from build123d import *

# Parameters (mm, degrees)
SKETCH_W        = 106.5
SKETCH_H        = 150
PAD_DEPTH       = 5
SKETCH001_W     = 5
SKETCH001_H     = 15.5
POCKET_DEPTH    = 5
FILLET_R        = 0.4
POCKET001_DEPTH = 5


with BuildPart() as part:
    # Sketch → Pad (new body)
    with BuildSketch(Plane.XY):
        Rectangle(SKETCH_W, SKETCH_H)
    extrude(amount=PAD_DEPTH)

    # Sketch001 (on Face6 of Pad) → Pocket (cut)
    with BuildSketch(Plane.XY.offset(5)):
        with Locations((-50.75, 67.25)):
            Rectangle(SKETCH001_W, SKETCH001_H)
        with Locations((50.75, 67.25)):
            Rectangle(SKETCH001_W, SKETCH001_H)
        with Locations((50.75, -67.25)):
            Rectangle(SKETCH001_W, SKETCH001_H)
        with Locations((-50.75, -67.25)):
            Rectangle(SKETCH001_W, SKETCH001_H)
    extrude(amount=-POCKET_DEPTH, mode=Mode.SUBTRACT)

    # Fillet
    fillet_edges = [part.edges().sort_by_distance(p)[0] for p in [
        (-48.25, 75, 2.5),
        (-48.25, 59.5, 2.5),
        (-53.25, 59.5, 2.5),
        (48.25, 75, 2.5),
        (48.25, 59.5, 2.5),
        (53.25, 59.5, 2.5),
        (53.25, -59.5, 2.5),
        (48.25, -59.5, 2.5),
        (48.25, -75, 2.5),
        (-48.25, -75, 2.5),
        (-48.25, -59.5, 2.5),
        (-53.25, -59.5, 2.5),
        (-48.25, 67.25, 5),
        (-50.75, 59.5, 5),
        (-53.25, 0, 5),
        (-50.75, -59.5, 5),
        (-48.25, -67.25, 5),
        (0, -75, 5),
        (48.25, -67.25, 5),
        (50.75, -59.5, 5),
        (53.25, 0, 5),
        (50.75, 59.5, 5),
        (48.25, 67.25, 5),
        (0, 75, 5),
    ]]
    fillet(fillet_edges, radius=FILLET_R)

    # Sketch002 (on Face29 of Fillet) → Pocket001 (cut)
    with BuildSketch(Plane.XY.offset(5)):
        with BuildLine():
            ThreePointArc((-40, -40), (-25, -55), (-10, -40))
            Line((-10, -40), (-10, 40))
            ThreePointArc((-10, 40), (-25, 55), (-40, 40))
            Line((-40, -40), (-40, 40))
        make_face()
        with BuildLine():
            ThreePointArc((10, -40), (25, -55), (40, -40))
            Line((40, -40), (40, 40))
            ThreePointArc((40, 40), (25, 55), (10, 40))
            Line((10, -40), (10, 40))
        make_face()
    extrude(amount=-POCKET001_DEPTH, mode=Mode.SUBTRACT)


solid = part.part
Design review of the part built by this model. Coordinates are the model's own, in mm. A direction names the side the tool comes from. Coordinates: 2 decimals unless noted, no trailing zeros. Order: outer loops, then holes, each group sorted by start corner. A loop starts at its lowest first (then second) coordinate and runs counter-clockwise, first axis right, second up.
Item 1: For faces 4 (the flat face through (48.25, 67, 2)), 5 (the flat face through (-48.25, 67, 2)), 6 (the flat face through (-10, -1, 3)), 7 (the flat face through (-51, -59.5, 2)), list the 3-axis set-ups (+Z, -Z, +X, -X, +Y, -Y) from which the entire face can be reached by the end or side of a thin tool; tool diameter is ignored.
Item 2: Take a section at A-A, the plane y = -16. Write out the cut boundary in (x, z), then the cut area to 3 significant figures.
Item 3: The part is to be moulded in two halves that separate along X. For faces 1 (the flat face through (-53.25, -1, 2)), 2 (the cylindrical face through (25, 55, 3)), 3 (the flat face through (-1, 75, 2)), say which applies: pulls with the +X half, pulls with the -X half, needs draft (parallel to the pull), parting line crosses it, or undercut.
Item 4: Take a section at B-B, the plane x = 25. Write out the cut boundary in (y, z).
Item 5: For pin 1 Ø2 at (x, z) = (50, 1) entering from +Y; pin 2 Ø2.5 at (y, z) = (66.5, 3) entering from +X; pin 3 Ø1.3 at (x, z) = (51, 1) entering from -Y, all flat-tipped, find the tip position at first contact; note any pin that passes through.
Item 6: Take a section at C-C, the plane z = 1.2. Count the separate pieces of the cut face and the enclosed holes in it, then the cut area to 3 significant figures.
Item 7: For line 1 (X direction, y = 36, z = 4.4); line 2 (X direction, y = 45.5, z = 2.2); line 3 (Y direction, x = 26, z = 4), list the stretches that pass through material, from the lowest coordinate up.
Item 8: Take a section at D-D, the plane x = -31.5. Write out the cut boundary in (y, z), then the cut area to 3 significant figures.
The answers:
1. face 4: +Z, -Z, +X, +Y
1. face 5: +Z, -Z, -X, +Y
1. face 6: +Z, -Z
1. face 7: +Z, -Z, -X, -Y
2. outline: (-53.25, 0) - (-40, 0) - (-40, 5) - (-52.85, 5) arc R0.4 ccw to (-53.25, 4.6) - close; (-10, 0) - (10, 0) - (10, 5) - (-10, 5) - close; (40, 0) - (53.25, 0) - (53.25, 4.6) arc R0.4 ccw to (52.85, 5) - (40, 5) - close
2. area: 232 mm2
3. face 1: pulls with the -X half
3. face 2: undercut
3. face 3: needs draft
4. outline: (-75, 0) - (-55, 0) - (-55, 5) - (-74.6, 5) arc R0.4 ccw to (-75, 4.6) - close; (55, 0) - (75, 0) - (75, 4.6) arc R0.4 ccw to (74.6, 5) - (55, 5) - close
5. pin 1: stops at y = 59.5
5. pin 2: stops at x = 48.25
5. pin 3: stops at y = -59.5
6. separate pieces: 1
6. enclosed holes: 2
6. area: 9,450 mm2
7. line 1: x = -53.25 to -40, -10 to 10, 40 to 53.25
7. line 2: x = -53.25 to -38.96, -11.04 to 11.04, 38.96 to 53.25
7. line 3: y = -75 to -54.97, 54.97 to 75
8. outline: (-75, 0) - (-53.52, 0) - (-53.52, 5) - (-74.6, 5) arc R0.4 ccw to (-75, 4.6) - close; (53.52, 0) - (75, 0) - (75, 4.6) arc R0.4 ccw to (74.6, 5) - (53.52, 5) - close
8. area: 215 mm2
